from build123d import *

# Parameters (mm, degrees)
BOSS_EXTRUDE1_DEPTH = 8
SKETCH2_R           = 1.6
CUT_EXTRUDE1_DEPTH  = 37.084183


with BuildPart() as part:
    # Sketch1 → Boss-Extrude1 (new body)
    with BuildSketch(Plane(origin=(0, 0, 0), x_dir=(1, 0, 0), z_dir=(0, 1, 0))):
        with BuildLine():
            Line((-20.5, 27.5), (20.5, 27.5))
            ThreePointArc((20.5, 27.5), (25.449747468, 25.449747468), (27.5, 20.5))
            Line((27.5, 20.5), (27.5, 11.5841835))
            Line((27.5, 11.5841835), (37.5, 11.5841835))
            Line((37.5, 11.5841835), (37.5, 9.5841835))
            Line((37.5, 9.5841835), (27.5, 9.5841835))
            Line((27.5, 9.5841835), (25.5, 9.5841835))
            Line((25.5, 9.5841835), (25.5, 20.5))
            ThreePointArc((25.5, 20.5), (24.035533906, 24.035533906), (20.5, 25.5))
            Line((20.5, 25.5), (-20.5, 25.5))
            ThreePointArc((-20.5, 25.5), (-24.035533906, 24.035533906), (-25.5, 20.5))
            Line((-25.5, 20.5), (-25.5, -20.5))
            ThreePointArc((-25.5, -20.5), (-24.035533906, -24.035533906), (-20.5, -25.5))
            Line((-20.5, -25.5), (20.5, -25.5))
            ThreePointArc((20.5, -25.5), (24.035533906, -24.035533906), (25.5, -20.5))
            Line((25.5, -20.5), (25.5, -6.177954833))
            Line((25.5, -6.177954833), (27.5, -6.177954833))
            Line((27.5, -6.177954833), (37.5, -6.177954833))
            Line((37.5, -6.177954833), (37.5, -8.177954833))
            Line((37.5, -8.177954833), (27.5, -8.177954833))
            Line((27.5, -8.177954833), (27.5, -20.5))
            ThreePointArc((27.5, -20.5), (25.449747468, -25.449747468), (20.5, -27.5))
            Line((20.5, -27.5), (-20.5, -27.5))
            ThreePointArc((-20.5, -27.5), (-25.449747468, -25.449747468), (-27.5, -20.5))
            Line((-27.5, -20.5), (-27.5, 20.5))
            ThreePointArc((-27.5, 20.5), (-25.449747468, 25.449747468), (-20.5, 27.5))
        make_face()
    extrude(amount=BOSS_EXTRUDE1_DEPTH)

    # Sketch2 → Cut-Extrude1 (cut)
    with BuildSketch(Plane(origin=(0, 0, -11.5841835), x_dir=(-1, 0, 0), z_dir=(0, 0, -1))):
        with Locations((-32.5, 4)):
            Circle(SKETCH2_R)
    extrude(amount=-CUT_EXTRUDE1_DEPTH, mode=Mode.SUBTRACT)


solid = part.part
Build history of the part. All positions in model axes, mm. A direction names the side the tool comes from. Give positions to 0.01 mm unless a question says otherwise; leave off trailing zeros. Order: outer loops, then holes, each group sorted by start corner. A loop starts at its lowest first (then second) coordinate and runs counter-clockwise, first axis right, second up. Notation, with made-up numbers: M -25.75,42.5 L -14.75,42.5 A10 cw -14.75,52.5 Z; hole C 52.25,19 d6. An arc over 180 degrees is marked long. Put each result on its own line as item: value.
Item 1: Cut at C-C on z = -13. Write the cut outline in (x, y).
Results are:
outline: M -27.5,0 L -25.5,0 L -25.5,8 L -27.5,8 Z; M 25.5,0 L 27.5,0 L 27.5,8 L 25.5,8 Z
Item 2: Cut at D-D on x = 32.5. Write the cut outline in (y, z), then the cut area to 3 significant figures.
Results are:
outline: M 0,-11.58 L 2.4,-11.58 L 2.4,-9.58 L 0,-9.58 Z; M 0,6.18 L 2.4,6.18 L 2.4,8.18 L 0,8.18 Z; M 5.6,-11.58 L 8,-11.58 L 8,-9.58 L 5.6,-9.58 Z; M 5.6,6.18 L 8,6.18 L 8,8.18 L 5.6,8.18 Z
area: 19.2 mm2
Item 3: Cut at B-B on x = -5.5. Write the cut outline in (y, z), then the cut area to 3 significant figures.
Results are:
outline: M 0,-27.5 L 8,-27.5 L 8,-25.5 L 0,-25.5 Z; M 0,25.5 L 8,25.5 L 8,27.5 L 0,27.5 Z
area: 32.0 mm2
Item 4: Cut at A-A on y = 4. Count the separate pieces of the cut face and the enclosed holes in it, then the cut area to 3 significant figures.
Results are:
separate pieces: 3
enclosed holes: 0
area: 399 mm2
Item 5: Pull direction Z, two halves, no side cores. Call faces 5 (the face through (-24, 3.94, -24.07)), 6 (the face through (25.4, 3.9, -25.5)), 7 (the face through (37.5, 4, -11)): +Z half, -Z half, draft (parallel to the pull), parting line (faces both ways), or undercut.
Results are:
face 5: undercut
face 6: -Z half
face 7: draft
Item 6: Drop flat-ended pins along their axis: pin 1 Ø10 at (x, z) = (23, 21.5) entering from +Y; pin 2 Ø1.9 at (x, y) = (32.5, 4) entering from -Z; pin 3 Ø4 at (y, z) = (4.5, 13) entering from +X; pin 4 Ø2.5 at (x, y) = (31, 6) entering from +Z. Give the stop position or say it passes through.
Results are:
pin 1: y = 8
pin 2: through
pin 3: x = 27.5
pin 4: z = 8.18
Item 7: Which spindle directions (+Z, -Z, +X, -X, +Y, -Y) get a long thin tool onto all of the face, cutting with end or side? Do faces 1 (the face through (34.1, 4.07, 7.16)), 2 (the face through (33, 6, 8.178)), 3 (the face through (32, 6, -11.584)), 4 (the face through (24, 3.94, 24.07)). Say none if no direction does.
Results are:
face 1: +Z, -Z
face 2: +Z, +X, +Y, -Y
face 3: -Z, +X, +Y, -Y
face 4: +Y, -Y
Item 8: Wall check: probe 1 along X at (y, z) = (5, -14); probe 2 along Z at (x, y) = (30.5, 5.5); probe 3 along Y at (x, z) = (32.5, -10.55). Give the ranges that are in metal, low to high.
Results are:
probe 1: -27.5 to -25.5, 25.5 to 27.5
probe 2: -11.58 to -9.58, 6.18 to 8.18
probe 3: 0 to 2.4, 5.6 to 8
